Input: part model. Units: mm. Frame: model coordinates. Face numbers are marked on the shaded views. A direction names the side the tool comes from. Round coordinates to 2 decimals unless told otherwise and drop trailing zeros. Write each loop counter-clockwise with the first axis right and the second up, starting at its lowest first coordinate (ties: lowest second). Pieces come first, ordered by that corner, then holes. Notation, with made-up numbers: (18.25, 38) - (40.25, 38) arc R16 cw to (40.25, 65) - close; hole circle Ø3 at (2.25, -16.75). An arc over 180 degrees is marked (long way). Use one line per item in the form item = value.
```python
from build123d import *

# Parameters (mm, degrees)
F0_R     = 9.525
F0_R_2   = 6.35
F1_DEPTH = 12.7
F2_R     = 12.7
F3_DEPTH = 101.6
F4_R     = 9.525
F4_R_2   = 6.35
F5_DEPTH = 25.4


with BuildPart() as f1:
    # F0 (on Front) → F1 (new body)
    with BuildSketch(Plane.XZ):
        Circle(F0_R)
        Circle(F0_R_2, mode=Mode.SUBTRACT)
    extrude(amount=F1_DEPTH)

    # F2 (on face) → F3 (join)
    with BuildSketch(Plane.XZ.offset(12.7)):
        Circle(F2_R)
    extrude(amount=F3_DEPTH)

    # F4 (on face) → F5 (join)
    with BuildSketch(Plane.XZ.offset(114.3)):
        Circle(F4_R)
        Circle(F4_R_2, mode=Mode.SUBTRACT)
    extrude(amount=F5_DEPTH)


solid = f1.part
```
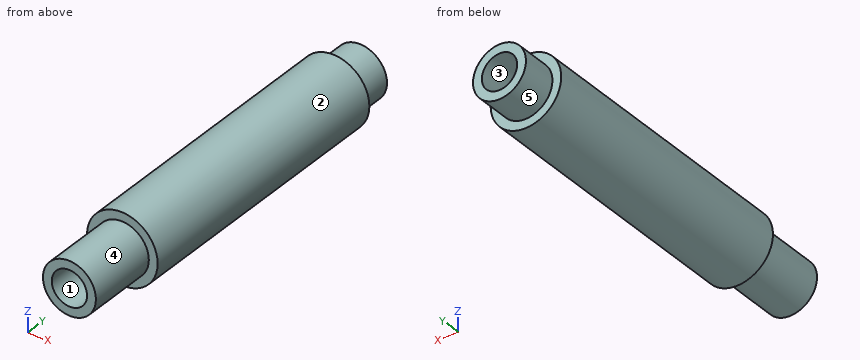
(1) Cut plane D-D on z = 11. Output: boundary loops of the cut face in (x, y), then the cut area to 3 significant figures.
Derived:
outline = (-6.35, -114.3) - (6.35, -114.3) - (6.35, -12.7) - (-6.35, -12.7) - close
area = 1,290 mm^2
(2) Cut plane B-B on z = 0. Output: boundary loops of the cut face in (x, y) (3 decimals), then the cut area to 3 significant figures.
Derived:
outline = (-12.7, -114.3) - (-9.525, -114.3) - (-9.525, -139.7) - (-6.35, -139.7) - (-6.35, -114.3) - (6.35, -114.3) - (6.35, -139.7) - (9.525, -139.7) - (9.525, -114.3) - (12.7, -114.3) - (12.7, -12.7) - (9.525, -12.7) - (9.525, 0) - (6.35, 0) - (6.35, -12.7) - (-6.35, -12.7) - (-6.35, 0) - (-9.525, 0) - (-9.525, -12.7) - (-12.7, -12.7) - close
area = 2,820 mm^2
(3) Cut plane A-A on x = 0. Output: boundary loops of the cut face in (y, z) (3 decimals).
Derived:
outline = (-139.7, -9.525) - (-114.3, -9.525) - (-114.3, -12.7) - (-12.7, -12.7) - (-12.7, -9.525) - (0, -9.525) - (0, -6.35) - (-12.7, -6.35) - (-12.7, 6.35) - (0, 6.35) - (0, 9.525) - (-12.7, 9.525) - (-12.7, 12.7) - (-114.3, 12.7) - (-114.3, 9.525) - (-139.7, 9.525) - (-139.7, 6.35) - (-114.3, 6.35) - (-114.3, -6.35) - (-139.7, -6.35) - close
(4) Material intervals for L1, parallel to Z at x = 0, y = -131 (3 decimals); L2, parallel to Y at x = 0.25, z = -1; L3, parallel to Z at x = 0.5, y = -31, sorted ascending.
Derived:
L1 = -9.525 to -6.35, 6.35 to 9.525
L2 = -114.3 to -12.7
L3 = -12.69 to 12.69
(5) Cut plane C-C on y = -14.5. Output: boundary loops of the cut face in (x, z).
Derived:
outline = circle Ø25.4 at (0, 0)
(6) Draft query along X for the marked faces 1, 2 and 3. Return one class per face: released by +X, released by -X, zero draft, split by the parting line, or undercut.
Derived:
face_1 = undercut
face_2 = split by the parting line
face_3 = undercut
(7) Access query for the marked faces 4 and 5. Directions: +Z, -Z, +X, -X, +Y, -Y. A direction counts if a zero-diameter tool reaches every point of the face in a straight line with its end or side. Return the directions, or none.
Derived:
face_4 = -Y
face_5 = +Y
(8) First-contact query: pin 1 Ø10 at (y, z) = (-92.5, -10) entering from +X; pin 2 Ø3 at (x, y) = (4, -55) entering from +Z; pin 3 Ø10 at (x, z) = (0, 0) entering from -Y; pin 4 Ø7.5 at (x, z) = (4.5, 0) entering from -Y. Flat tips, straight axial feed; report the tip coordinate or a pass-through.
Derived:
pin_1 = 11.67
pin_2 = 12.45
pin_3 = -114.3
pin_4 = -139.7
